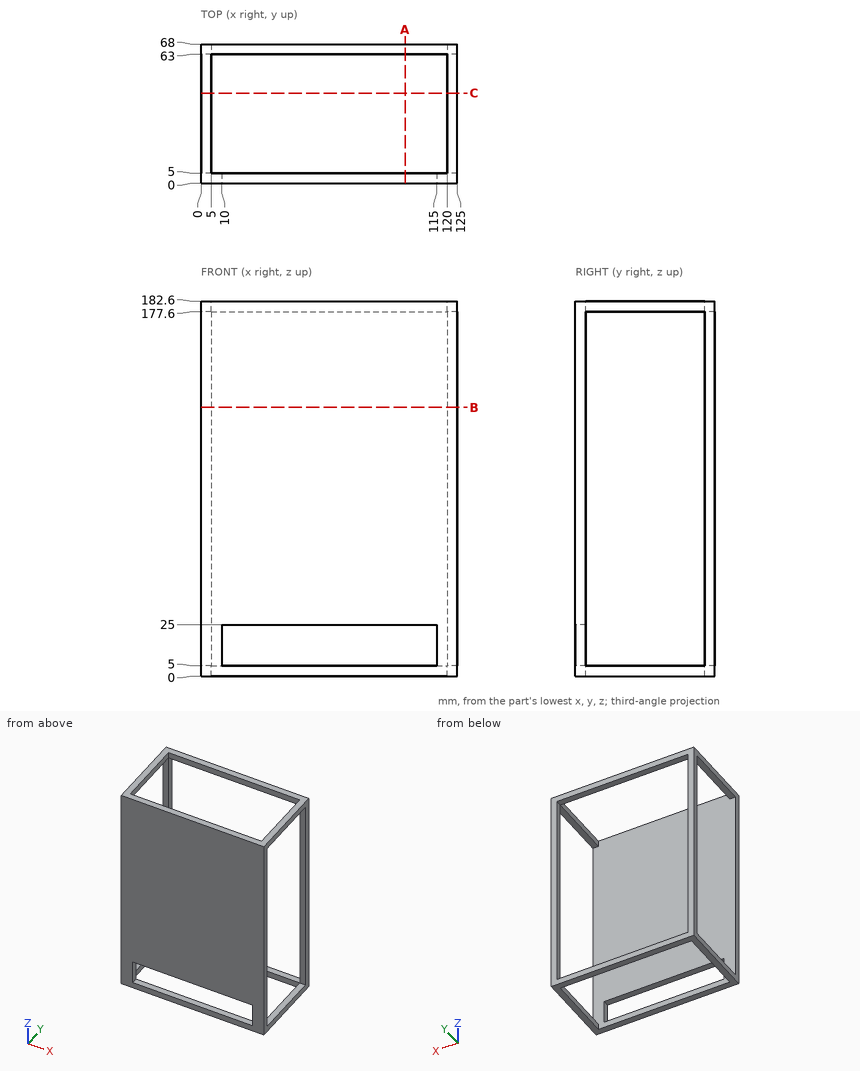
Can you work these out from the drawing? Everything is in mm from the part's minimum corner. Give positions to 0.01 mm unless a question says otherwise; leave off trailing zeros. Loops run counter-clockwise (first coordinate to the right, second up) from the corner with the lowest first, then second, coordinate; pieces in that order, holes last. Notation, with made-up numbers: (66.25, 23) -> (86.25, 23) arc R18 ccw to (86.25, 36) -> close; hole circle Ø11 at (65, 6). An arc over 180 degrees is marked (long way). Return JSON: item names as keys, results as strings.
Q1. I need wall thicknesses on probe 1 along X at (y, z) = (64, 109.5); probe 2 along Z at (x, y) = (30, 64); probe 3 along Y at (x, z) = (60, 157). Which ranges of each line are inside material? Lowest first, please.
Checks:
{"probe 1": "x = 0 to 5, 120 to 125", "probe 2": "z = 0 to 5, 177.6 to 182.6", "probe 3": "y = 0 to 5"}
Q2. For pin 1 Ø5.5 at (x, y) = (85, 64.5) entering from -Z; pin 2 Ø6 at (x, z) = (40.5, 21.5) entering from +Y; pin 3 Ø8 at (x, z) = (17, 56.5) entering from +Y, each with a flat end and sliding along its axis, tell me the tip position at first contact or that it passes through.
Checks:
{"pin 1": "stops at z = 0", "pin 2": "passes through", "pin 3": "stops at y = 5"}
Q3. I want a section at C-C, the plane y = 44. List the corners of the cut face in (x, z) for me, then the cut area to 3 significant figures.
Checks:
{"outline": "(0, 0) -> (5, 0) -> (5, 5) -> (0, 5) -> close; (0, 177.6) -> (5, 177.6) -> (5, 182.6) -> (0, 182.6) -> close; (120, 0) -> (125, 0) -> (125, 5) -> (120, 5) -> close; (120, 177.6) -> (125, 177.6) -> (125, 182.6) -> (120, 182.6) -> close", "area": "100 mm2"}
Q4. I want a section at B-B, the plane z = 131. List the corners of the cut face in (x, y) for me, then the cut area to 3 significant figures.
Checks:
{"outline": "(0, 0) -> (125, 0) -> (125, 5) -> (0, 5) -> close; (0, 63) -> (5, 63) -> (5, 68) -> (0, 68) -> close; (120, 63) -> (125, 63) -> (125, 68) -> (120, 68) -> close", "area": "675 mm2"}
Q5. I want a section at A-A, the plane x = 99.5. List the corners of the cut face in (y, z) for me, then the cut area to 3 significant figures.
Checks:
{"outline": "(0, 0) -> (5, 0) -> (5, 5) -> (0, 5) -> close; (0, 25) -> (5, 25) -> (5, 182.6) -> (0, 182.6) -> close; (63, 0) -> (68, 0) -> (68, 5) -> (63, 5) -> close; (63, 177.6) -> (68, 177.6) -> (68, 182.6) -> (63, 182.6) -> close", "area": "863 mm2"}
